Source: CAD feature listing. Evaluate the final solid. Frame: model axes, mm. A direction names the side the tool comes from. Give positions to 0.01 mm unless a question says otherwise; leave off trailing zeros. Loops run counter-clockwise (first coordinate to the right, second up) from the corner with the lowest first, then second, coordinate; pieces in that order, holes last. Notation, with made-up numbers: (-15, -22.5) -> (10, -22.5) arc R21 cw to (10, -16.5) -> close; hole circle Ø11 at (7.25, -28). An arc over 180 degrees is marked (long way). Return JSON: item names as keys, results as strings. Group by question number.
(1) Cut plane C-C on y = -2.5. Return loops of the section in (x, z) (3 decimals).
(2) Pin query (flat end, axial travel): pin 1 (1 mm diameter, centred on x = 20.5, z = 35.5, fed in from -Y). Return the tip coordinate at first contact, or that it passes through.
(3) Ray query, line 1 (X direction, y = -5.25, z = 45) (3 decimals); line 2 (X direction, y = -0.5, z = 19.5) (3 decimals); line 3 (Z direction, x = 19, y = -2). Return the intervals inside material, ascending. Write a range as from..to.
(4) Cut plane A-A on z = 5. Return loops of the section in (x, y) (3 decimals).
(5) Cut plane B-B on x = 5. Return loops of the section in (y, z) (3 decimals).
(6) Draft query along X for faces 3 (the face through (9, 0, 25)), 4 (the face through (0, -4, 25)), 5 (the face through (23.625, -4, 25)), 6 (the face through (11.375, -4, 25)). Return one class per face: released by +X, released by -X, zero draft, split by the parting line, or undercut.
(7) Cut plane D-D on z = 32.5. Return loops of the section in (x, y) (3 decimals).
(8) Access query for faces 1 (the face through (17, -4, 36.5)), 2 (the face through (17, -4, 0)). Directions: +Z, -Z, +X, -X, +Y, -Y. A direction counts if a zero-diameter tool reaches every point of the face in a straight line with its end or side. Return the directions, or none.
```python
from build123d import *

# Parameters (mm, degrees)
SKETCH_1_W          = 35
SKETCH_1_H          = 50
SKETCH_1_W_2        = 12.25
SKETCH_1_H_2        = 23
EXTRUDE_2_DEPTH     = 7.5
SKETCH_2_R          = 1.525
CUT_EXTRUDE_1_DEPTH = 62.491869381


with BuildPart() as part:
    # 草图1 → 凸台-拉伸2 (new body)
    with BuildSketch(Plane(origin=(0, 0, 0), x_dir=(1, 0, 0), z_dir=(0, 1, 0))):
        with Locations((17.5, -25)):
            Rectangle(SKETCH_1_W, SKETCH_1_H)
        with Locations((17.5, -25)):
            Rectangle(SKETCH_1_W_2, SKETCH_1_H_2, mode=Mode.SUBTRACT)
    extrude(amount=-EXTRUDE_2_DEPTH)

    # 草图2 → 切除-拉伸1 (cut, through all)
    with BuildSketch(Plane.XZ.offset(7.5)):
        with Locations(Location((5, 5, 0), (0, 0, 270))):
            Circle(SKETCH_2_R)
        with Locations(Location((5, 45, 0), (0, 0, 90))):
            Circle(SKETCH_2_R)
        with Locations(Location((30, 45, 0), (0, 0, 270))):
            Circle(SKETCH_2_R)
        with Locations(Location((30, 5, 0), (0, 0, 90))):
            Circle(SKETCH_2_R)
    extrude(amount=-CUT_EXTRUDE_1_DEPTH, mode=Mode.SUBTRACT)


solid = part.part
```
Answers:
{
 "1": {"outline": "(0, 0) -> (35, 0) -> (35, 50) -> (0, 50) -> close; hole circle Ø3.05 at (5, 5); hole circle Ø3.05 at (5, 45); hole (11.375, 13.5) -> (23.625, 13.5) -> (23.625, 36.5) -> (11.375, 36.5) -> close; hole circle Ø3.05 at (30, 5); hole circle Ø3.05 at (30, 45)"},
 "2": {"pin 1": "through"},
 "3": {"line 1": "0..3.475, 6.525..28.475, 31.525..35", "line 2": "0..11.375, 23.625..35", "line 3": "0..13.5, 36.5..50"},
 "4": {"outline": "(0, -7.5) -> (3.475, -7.5) -> (3.475, 0) -> (0, 0) -> close; (6.525, -7.5) -> (28.475, -7.5) -> (28.475, 0) -> (6.525, 0) -> close; (31.525, -7.5) -> (35, -7.5) -> (35, 0) -> (31.525, 0) -> close"},
 "5": {"outline": "(-7.5, 0) -> (0, 0) -> (0, 3.475) -> (-7.5, 3.475) -> close; (-7.5, 6.525) -> (0, 6.525) -> (0, 43.475) -> (-7.5, 43.475) -> close; (-7.5, 46.525) -> (0, 46.525) -> (0, 50) -> (-7.5, 50) -> close"},
 "6": {"face 3": "zero draft", "face 4": "released by -X", "face 5": "undercut", "face 6": "undercut"},
 "7": {"outline": "(0, -7.5) -> (11.375, -7.5) -> (11.375, 0) -> (0, 0) -> close; (23.625, -7.5) -> (35, -7.5) -> (35, 0) -> (23.625, 0) -> close"},
 "8": {"face 1": "+Y, -Y", "face 2": "-Z, +X, -X, +Y, -Y"}
}
